Could you check a few things on this model? Use its own coordinates, in mm. Face numbers are marked on the shaded views. Give positions to 0.01 mm unless a question says otherwise; leave off trailing zeros. Write each loop counter-clockwise with the first axis right and the second up, starting at its lowest first coordinate (ties: lowest second). Pieces come first, ordered by that corner, then holes. Notation, with made-up numbers: M 52.25,52.25 L 96.25,52.25 A26 ccw 96.25,66.25 Z; hole C 38.25,-30 d7. An arc over 180 degrees is marked long. Use one line per item in the form item = value.
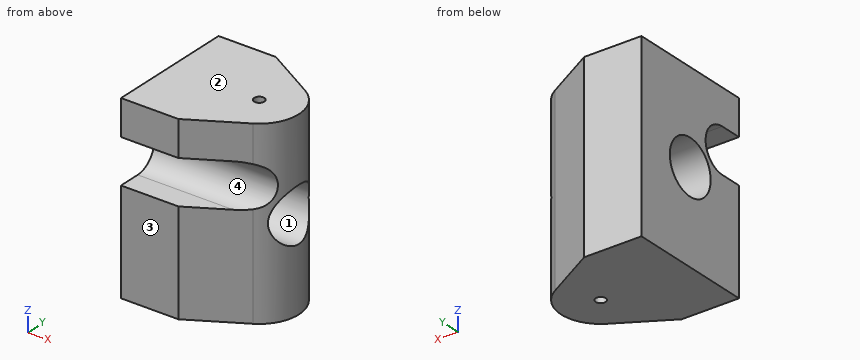
from build123d import *

# Parameters (mm, degrees)
ESQUISSE2_R      = 3.25
EXTRUSION1_DEPTH = 57.5
ESQUISSE5_R      = 17
EXTRUSION3_DEPTH = 108.688718072


with BuildPart() as part:
    # Esquisse2 → Extrusion1 (new, symmetric)
    with BuildSketch(Plane.XY):
        with BuildLine():
            Line((-56.5, 40.6), (-56.5, -40.6))
            Line((-56.5, -40.6), (-20.321262787, -40.6))
            Line((-20.321262787, -40.6), (12.5, -21.650635095))
            ThreePointArc((12.5, -21.650635095), (25, 0), (12.5, 21.650635095))
            Line((12.5, 21.650635095), (-20.321262787, 40.6))
            Line((-20.321262787, 40.6), (-56.5, 40.6))
        make_face()
        Circle(ESQUISSE2_R, mode=Mode.SUBTRACT)
    extrude(amount=EXTRUSION1_DEPTH, both=True)

    # Esquisse5 → Extrusion3 (cut, through all)
    with BuildSketch(Plane.ZY.offset(56.5)):
        Circle(ESQUISSE5_R)
        with BuildLine():
            Line((7.3, -40.6), (7.3, -26.7))
            ThreePointArc((7.3, -26.7), (21.2, -12.8), (35.1, -26.7))
            Line((35.1, -26.7), (35.1, -40.6))
            Line((35.1, -40.6), (7.3, -40.6))
        make_face()
    extrude(amount=-EXTRUSION3_DEPTH, mode=Mode.SUBTRACT)


solid = part.part
1) I want a section at A-A, the plane z = 48.5. Please give me the cut outline in (x, y), plus the area to 3 significant figures.
Checked values:
outline = M -56.5,-40.6 L -20.32,-40.6 L 12.5,-21.65 A25 ccw 12.5,21.65 L -20.32,40.6 L -56.5,40.6 Z; hole C 0,0 d6.5
area = 5,330 mm2
2) If I drill on L1, parallel to X at y = 0, z = 29; L2, parallel to Z at x = -35, y = -26; L3, parallel to Y at x = -34, z = 0, over which ranges is the centre line in solid material (lowest first)?
Checked values:
L1 = -56.5 to -3.25, 3.25 to 25
L2 = -57.5 to 7.32, 35.08 to 57.5
L3 = -40.6 to -17, 17 to 40.6
3) I want a section at B-B, the plane y = 0. Please give me the cut outline in (x, z).
Checked values:
outline = M -56.5,-57.5 L -3.25,-57.5 L -3.25,-17 L -56.5,-17 Z; M -56.5,17 L -3.25,17 L -3.25,57.5 L -56.5,57.5 Z; M 3.25,-57.5 L 25,-57.5 L 25,-17 L 3.25,-17 Z; M 3.25,17 L 25,17 L 25,57.5 L 3.25,57.5 Z
4) I want a section at D-D, the plane z = 0. Please give me the cut outline in (x, y).
Checked values:
outline = M -56.5,-40.6 L -20.32,-40.6 L 12.5,-21.65 A25 ccw 18.33,-17 L -56.5,-17 Z; M -56.5,17 L 18.33,17 A25 ccw 12.5,21.65 L -20.32,40.6 L -56.5,40.6 Z
5) Thinking about a two-plate mould opening in Z: for the marked faces 1, 2, 3 and 4, which applies, released by +Z, released by -Z, zero draft, split by the parting line, or undercut?
Checked values:
face_1 = undercut
face_2 = released by +Z
face_3 = zero draft
face_4 = undercut
6) For pin 1 Ø8.5 at (x, y) = (0, 0) entering from +Z; pin 2 Ø8 at (x, z) = (1.5, 20) entering from +Y; pin 3 Ø6 at (x, z) = (-16, -10.5) entering from -Y; pin 4 Ø4 at (x, y) = (0, 0) entering from -Z, each with a flat end and sliding along its axis, tell me the tip position at first contact or that it passes through.
Checked values:
pin_1 = 57.5
pin_2 = 30.31
pin_3 = -39.84
pin_4 = through
7) I want a section at C-C, the plane x = -31.5. Please give me the cut outline in (y, z), plus the area to 3 significant figures.
Checked values:
outline = M -40.6,-57.5 L 40.6,-57.5 L 40.6,57.5 L -40.6,57.5 L -40.6,35.1 L -26.7,35.1 A13.9 cw -26.7,7.3 L -40.6,7.3 Z; hole C 0,0 d34
area = 7,740 mm2
